Autodesk Inventor part; units mm, degrees
ref_plane "YZ Plane" through (0, 0, 0) normal (1, 0, 0) x (0, 1, 0)
ref_plane "XZ Plane" through (0, 0, 0) normal (0, 1, 0) x (-1, 0, 0)
ref_plane "XY Plane" through (0, 0, 0) normal (0, 0, 1) x (1, 0, 0)
sketch "Эскиз1" plane through (0, 0, 0) normal (0, 0, 1) x (1, 0, 0)
  line L0 (0, 0) -> (0, 64) construction
  line L1 (0, 64) -> (-15, 64)
  line L2 (-15, 64) -> (-15, 68)
  line L3 (-15, 68) -> (-35, 68)
  line L4 (-35, 68) -> (-35, 64)
  line L5 (-35, 64) -> (-49, 64)
  line L6 (-49, 64) -> (-49, 49)
  line L7 (-49, 49) -> (-53, 49)
  line L8 (-53, 49) -> (-53, 19)
  line L9 (-53, 19) -> (-49, 19)
  line L10 (-49, 19) -> (-49, 0)
  line L11 (-39, 22) -> (-39, 54)
  line L12 (0, 0) -> (-15, 0)
  line L13 (-15, 0) -> (-15, 4)
  line L14 (-15, 4) -> (-35, 4)
  line L15 (-35, 4) -> (-35, 0)
  line L16 (-35, 0) -> (-49, 0)
  line L17 (-39, 22) -> (-30, 22)
  line L18 (-30, 22) -> (-30, 18)
  line L19 (-30, 18) -> (-10, 18)
  line L20 (-10, 18) -> (-10, 22)
  line L21 (-10, 22) -> (0, 22)
  line L22 (-39, 54) -> (0, 54)
  line L23 (0, 64) -> (15, 64)
  line L24 (15, 64) -> (15, 68)
  line L25 (15, 68) -> (35, 68)
  line L26 (35, 68) -> (35, 64)
  line L27 (35, 64) -> (49, 64)
  line L28 (49, 64) -> (49, 49)
  line L29 (49, 49) -> (53, 49)
  line L30 (53, 49) -> (53, 19)
  line L31 (53, 19) -> (49, 19)
  line L32 (49, 19) -> (49, 0)
  line L33 (39, 22) -> (39, 54)
  line L34 (0, 0) -> (15, 0)
  line L35 (15, 0) -> (15, 4)
  line L36 (15, 4) -> (35, 4)
  line L37 (35, 4) -> (35, 0)
  line L38 (35, 0) -> (49, 0)
  line L39 (39, 22) -> (30, 22)
  line L40 (30, 22) -> (30, 18)
  line L41 (30, 18) -> (10, 18)
  line L42 (10, 18) -> (10, 22)
  line L43 (10, 22) -> (0, 22)
  line L44 (39, 54) -> (0, 54)
  point P0 (0, 32)
  point P1 (53, 32)
  dimension "d0" = 30
  dimension "d8" = 10
  dimension "d12" = 4
  dimension "d13" = 18
  dimension "d14" = 20
  dimension "d15" = 20
  dimension "d16" = 68
  dimension "d17" = 30
  dimension "d18" = 20
  dimension "d19" = 10
  dimension "d20" = 78
  dimension "d21" = 30
  dimension "d22" = 20
  dimension "d23" = 19
extrude "Выдавливание1" add sketch "Эскиз1" along normal blind 4
fillet "Сопряжение1" radius 8 2 edges at (-39, 54, 2) (39, 54, 2)
sketch "Эскиз2" plane through (0, 0, 4) normal (0, 0, 1) x (1, 0, 0)
  line L0 (0, 0) -> (0, 64)
  line L1 (15, 64) -> (-15, 64)
  line L2 (-49, 64) -> (-49, 49)
  line L3 (-35, 64) -> (-49, 64)
  point P0 (-44, 59)
  point P1 (-44, 27)
  point P2 (44, 59)
  point P3 (44, 27)
  dimension "d31" = 5
  dimension "d32" = 5
  dimension "d33" = 37
hole "Отверстие1" at (-44, 59, 4) at (-44, 27, 4) at (44, 59, 4) at (44, 27, 4) direction (0, 0, -1) diameter 2.8 depth 8
properties part number "stiffenerFront" material "Дерево (береза)"
CAD build for the part. Positions are in the model's coordinates, mm. A direction names the side the tool comes from. Round coordinates to 2 decimals unless told otherwise and drop trailing zeros. Write each loop counter-clockwise with the first axis right and the second up, starting at its lowest first coordinate (ties: lowest second). Pieces come first, ordered by that corner, then holes. Notation, with made-up numbers: (73, -39) - (91, -39) arc R36 ccw to (91, -5) - close; hole circle Ø4 at (12.5, 68). An arc over 180 degrees is marked (long way). Write item = value, one per line. Start each with the question number.
Q1. Mould opens along X. For faces 5 (the flat face through (-39, 34, 2)), 6 (the flat face through (-10, 20, 2)), 7 (the flat face through (-49, 57, 2)), 8 (the flat face through (-51, 19, 2)) say: pulls with the +X half, pulls with the -X half, needs draft (parallel to the pull), parting line crosses it, or undercut.
Q2. Drop flat-ended pins along their axis: pin 1 (1.5 mm diameter, centred on x = 39.5, z = 3.5, fed in from +Y); pin 2 (2 mm diameter, centred on y = 1.5, z = 2.5, fed in from +X); pin 3 (1.7 mm diameter, centred on x = 44, y = 27, fed in from -Z); pin 4 (1.2 mm diameter, centred on x = 50.5, z = 2.5, fed in from +Y). Give the stop position or say it passes through.
Q3. Band-saw the part on C-C (x = -44). Give the cut face in (y, z).
Q4. Probe L1, parallel to X at y = 27, z = 1.4; L2, parallel to Y at x = 44, z = 2.45; L3, parallel to X at y = 59, z = 0.95. List the from-to ranges inside material, lowest first. Write a range as from..to.
Q5. Band-saw the part on D-D (z = 2.65). Count the separate pieces of the cut face and the enclosed holes in it, then the cut area to 3 significant figures.
Q6. Band-saw the part on A-A (y = 32.5). Give the cut face in (x, z), then the cut area to 3 significant figures.
Q7. Band-saw the part on B-B (x = 26.5). Give the cut face in (y, z).
Q8. Which spindle directions (+Z, -Z, +X, -X, +Y, -Y) get a long thin tool onto all of the face, cutting with end or side? Do faces 1 (the flat face through (20, 18, 2)), 2 (the flat face through (-15, 2, 2)), 3 (the flat face through (-42, 0, 2)), 4 (the flat face through (-49, 10, 2)). Say none if no direction does.
Answers below:
q1.face_5 = undercut
q1.face_6 = undercut
q1.face_7 = pulls with the -X half
q1.face_8 = needs draft
q2.pin_1 = 64
q2.pin_2 = 49
q2.pin_3 = through
q2.pin_4 = 49
q3.outline = (0, 0) - (25.6, 0) - (25.6, 4) - (0, 4) - close; (28.4, 0) - (57.6, 0) - (57.6, 4) - (28.4, 4) - close; (60.4, 0) - (64, 0) - (64, 4) - (60.4, 4) - close
q4.L1 = -53..-45.4, -42.6..-39, 39..42.6, 45.4..53
q4.L2 = 0..25.6, 28.4..57.6, 60.4..64
q4.L3 = -49..-45.4, -42.6..42.6, 45.4..49
q5.separate_pieces = 1
q5.enclosed_holes = 5
q5.area = 3,860 mm2
q6.outline = (-53, 0) - (-39, 0) - (-39, 4) - (-53, 4) - close; (39, 0) - (53, 0) - (53, 4) - (39, 4) - close
q6.area = 112 mm2
q7.outline = (4, 0) - (18, 0) - (18, 4) - (4, 4) - close; (54, 0) - (68, 0) - (68, 4) - (54, 4) - close
q8.face_1 = +Z, -Z
q8.face_2 = +Z, -Z, -Y
q8.face_3 = +Z, -Z, +X, -X, -Y
q8.face_4 = +Z, -Z, -X, -Y
